from build123d import *

# Parameters (mm, degrees)
SKETCH1_W            = 70
SKETCH1_H            = 30
BOSS_EXTRUDE1_DEPTH  = 6.35
CUT_EXTRUDE1_DEPTH   = 54.400117041
CUT_EXTRUDE2_DEPTH   = 3.175
M3_CLEARANCE_HOLE2_D = 3.6
FILLET1_R            = 4
M3_CLEARANCE_HOLE3_D = 3.4


with BuildPart() as part:
    # Sketch1 → Boss-Extrude1 (new body)
    with BuildSketch(Plane.XZ):
        with Locations((-6.5, 18)):
            Rectangle(SKETCH1_W, SKETCH1_H)
    extrude(amount=-BOSS_EXTRUDE1_DEPTH)

    # Sketch9 → Cut-Extrude1 (cut, through all)
    with BuildSketch(Plane(origin=(0, 6.35, 0), x_dir=(1, 0, 0), z_dir=(0, 1, 0))):
        with BuildLine():
            Line((28.5, -12.1), (18.5, -12.1))
            ThreePointArc((18.5, -12.1), (13.949193338, -18), (18.5, -23.9))
            Line((18.5, -23.9), (28.5, -23.9))
            Line((28.5, -23.9), (28.5, -12.1))
        make_face()
    extrude(amount=-CUT_EXTRUDE1_DEPTH, mode=Mode.SUBTRACT)

    # Sketch10 → Cut-Extrude2 (cut)
    with BuildSketch(Plane(origin=(0, 6.35, 0), x_dir=(1, 0, 0), z_dir=(0, 1, 0))):
        with BuildLine():
            Line((28.5, -26.25), (20.049193338, -26.25))
            ThreePointArc((20.049193338, -26.25), (11.799193338, -18), (20.049193338, -9.75))
            Line((20.049193338, -9.75), (28.5, -9.75))
            Line((28.5, -9.75), (28.5, -26.25))
        make_face()
    extrude(amount=-CUT_EXTRUDE2_DEPTH, mode=Mode.SUBTRACT)

    # M3 Clearance Hole2 (through all)
    with Locations(Plane(origin=(-21.5, 6.35, 28), x_dir=(0, 0, 1), z_dir=(0, 1, 0))):
        with Locations((0, 0), (-20, 0), (-20, 20), (0, 20)):
            Hole(M3_CLEARANCE_HOLE2_D / 2)

    # Fillet1
    fillet1_edges = [part.edges().sort_by_distance(p)[0] for p in [
        (-41.5, 3.175, 33),
        (28.5, 3.175, 33),
        (28.5, 3.175, 3),
        (-41.5, 3.175, 3),
    ]]
    fillet(fillet1_edges, radius=FILLET1_R)

    # M3 Clearance Hole3 (through all)
    with Locations(Plane(origin=(-29, 6.35, 5.5), x_dir=(0, 0, 1), z_dir=(0, 1, 0))):
        with Locations((0, 0), (25, 0), (25, 35), (0, 35)):
            Hole(M3_CLEARANCE_HOLE3_D / 2)


solid = part.part
Design review of the part built by this model. Coordinates are the model's own, in mm. A direction names the side the tool comes from. Give positions to 0.01 mm unless a question says otherwise; leave off trailing zeros. Write each loop counter-clockwise with the first axis right and the second up, starting at its lowest first coordinate (ties: lowest second). Pieces come first, ordered by that corner, then holes. Notation, with made-up numbers: M 19.5,76 L 25.5,76 A30 ccw 25.5,106 Z; hole C -19,56.5 d2. An arc over 180 degrees is marked long. Return JSON: item names as keys, results as strings. Group by question number.
Item 1: Wall thickness on line 1 along X through (y, z) = (2.25, 8); line 2 along Z through (x, y) = (-20.5, 4.5); line 3 along X through (y, z) = (4, 7.5): over which ranges is each line inside the solid? List them lowest first.
Item 2: Take a section at D-D (z = 18). Give the boundary of the cut face in (x, y) (3 decimals).
Item 3: Take a section at B-B (z = 8). Give the boundary of the cut face in (x, y), plus the area to 3 significant figures.
Item 4: Take a section at C-C (y = 5.5). Count the separate pieces of the cut face and the enclosed holes in it, plus the area to 3 significant figures.
Item 5: Tool access review of faces 4 (the flat face through (19.6, 3.175, 24.1)), 5 (the flat face through (23, 2, 23.9)), 6 (the flat face through (-7, 3, 3)): name each direction out of +Z, -Z, +X, -X, +Y, -Y from which nothing blocks a thin tool from reaching the whole face with its end or side.
Item 6: The part is to be moulded in two halves that separate along X. For faces 1 (the flat face through (-41.5, 3, 18)), 2 (the cylindrical face through (-19.715, 3.131, 8.234)), 3 (the flat face through (-7, 3, 33)), say which applies: pulls with the +X half, pulls with the -X half, needs draft (parallel to the pull), parting line crosses it, or undercut.
Item 7: Clearance check with flat-ended pins moving along their axes: pin 1 Ø3.5 at (x, y) = (26, 1.5) entering from -Z; pin 2 Ø1.5 at (y, z) = (1, 30) entering from +X; pin 3 Ø8 at (x, z) = (20, 21.5) entering from +Y (3 decimals). State where each tip first meets the part, or that it passes through.
Item 8: Take a section at A-A (x = 6). Give the boundary of the cut face in (y, z).
Return value:
{
 "1": {"line 1": "x = -41.5 to -23.3, -19.7 to -3.3, 0.3 to 28.5", "line 2": "z = 3 to 6.5, 9.5 to 26.5, 29.5 to 33", "line 3": "x = -41.5 to -23.23, -19.77 to -3.23, 0.23 to 28.5"},
 "2": {"outline": "M -41.5,0 L 13.949,0 L 13.949,3.175 L 11.799,3.175 L 11.799,6.35 L -41.5,6.35 Z"},
 "3": {"outline": "M -41.5,0 L -23.3,0 L -23.3,6.35 L -41.5,6.35 Z; M -19.7,0 L -3.3,0 L -3.3,6.35 L -19.7,6.35 Z; M 0.3,0 L 28.5,0 L 28.5,6.35 L 0.3,6.35 Z", "area": "399 mm2"},
 "4": {"separate pieces": "1", "enclosed holes": "8", "area": "1,760 mm2"},
 "5": {"face 4": "+X, +Y", "face 5": "+X, +Y, -Y", "face 6": "-Z, +X, -X, +Y, -Y"},
 "6": {"face 1": "pulls with the -X half", "face 2": "undercut", "face 3": "needs draft"},
 "7": {"pin 1": "stops at z = 3", "pin 2": "stops at x = 28.49", "pin 3": "stops at y = 3.175"},
 "8": {"outline": "M 0,3 L 6.35,3 L 6.35,3.8 L 0,3.8 Z; M 0,7.2 L 6.35,7.2 L 6.35,28.8 L 0,28.8 Z; M 0,32.2 L 6.35,32.2 L 6.35,33 L 0,33 Z"}
}
